```python
from build123d import *

# Parameters (mm, degrees)
SKETCH1_R           = 29
SKETCH1_R_2         = 12
BOSS_EXTRUDE1_DEPTH = 8
CHAMFER1_SIZE       = 1
CHAMFER2_SIZE       = 1


with BuildPart() as part:
    # Sketch1 → Boss-Extrude1 (new body)
    with BuildSketch(Plane.XY):
        Circle(SKETCH1_R)
        Circle(SKETCH1_R_2, mode=Mode.SUBTRACT)
    extrude(amount=BOSS_EXTRUDE1_DEPTH)

    # Chamfer1
    chamfer1_edges = [part.edges().sort_by_distance(p)[0] for p in [
        (-12, 0, 0),
        (-12, 0, 8),
    ]]
    chamfer(chamfer1_edges, length=CHAMFER1_SIZE)

    # Chamfer2
    chamfer2_edges = [part.edges().sort_by_distance(p)[0] for p in [
        (-29, 0, 0),
        (-29, 0, 8),
    ]]
    chamfer(chamfer2_edges, length=CHAMFER2_SIZE)


solid = part.part
```
Work out the finished part from the listing and answer in its coordinate system (mm). Coordinates: 2 decimals unless noted, no trailing zeros. Write each loop counter-clockwise with the first axis right and the second up, starting at its lowest first coordinate (ties: lowest second). Pieces come first, ordered by that corner, then holes. Notation, with made-up numbers: (-15, -2) - (-5, -2) arc R25 ccw to (-5, 23) - close; hole circle Ø9 at (-17, 80). An arc over 180 degrees is marked (long way). Answer as a JSON object with one key per item and string values.
Q1. Consider L1, parallel to Y at x = 0, z = 3.8; L2, parallel to X at y = -1, z = 7.75; L3, parallel to Y at x = 8, z = 5.75. Determine where each line is inside the solid, lowest interval first. Write a range as from..to.
Results list:
{"L1": "y = -29..-12, 12..29", "L2": "x = -28.23..-12.71, 12.71..28.23", "L3": "y = -27.87..-8.94, 8.94..27.87"}
Q2. For a pull along Y with two mould halves and no side action, classify faces 1 (the cylindrical face through (-11.99, 0.53, 3.96)), 2 (the flat face through (6, -12, 8)), 3 (the cylindrical face through (13.38, -25.73, 3.96)) as pulls with the +Y half, pulls with the -Y half, needs draft (parallel to the pull), parting line crosses it, or undercut.
Results list:
{"face 1": "undercut", "face 2": "needs draft", "face 3": "parting line crosses it"}
Q3. Find section A-A (y = 0). Write down the section's boundary in (x, z).
Results list:
{"outline": "(-29, 1) - (-28, 0) - (-13, 0) - (-12, 1) - (-12, 7) - (-13, 8) - (-28, 8) - (-29, 7) - close; (12, 1) - (13, 0) - (28, 0) - (29, 1) - (29, 7) - (28, 8) - (13, 8) - (12, 7) - close"}
Q4. Given pin 1 Ø1 at (x, y) = (-18.5, -5.5) entering from -Z; pin 2 Ø19 at (x, y) = (0, 0) entering from +Z; pin 3 Ø2 at (y, z) = (-1.5, 1) entering from +X; pin 4 Ø1.5 at (x, z) = (12, 6.5) entering from -Y, each flat-ended and moving along its own axis, determine where each tip first touches the part or whether it passes through.
Results list:
{"pin 1": "stops at z = 0", "pin 2": "passes through", "pin 3": "stops at x = 29", "pin 4": "stops at y = -26.73"}
Q5. Find section C-C (z = 3). Write down the section's boundary in (x, y), plus the area to 3 significant figures.
Results list:
{"outline": "circle Ø58 at (0, 0); hole circle Ø24 at (0, 0)", "area": "2,190 mm^2"}
